Read the model definition and answer for the solid it produces. Units are mm, in the model's axes. Face numbers are marked on the shaded views. Coordinates: 2 decimals unless noted, no trailing zeros. Order: outer loops, then holes, each group sorted by start corner. A loop starts at its lowest first (then second) coordinate and runs counter-clockwise, first axis right, second up. Notation, with made-up numbers: (-2.5, -11.5) -> (2.5, -11.5) arc R10 ccw to (2.5, 3.5) -> close; hole circle Ø6 at (-18.5, 44.25). An arc over 180 degrees is marked (long way). Answer in a Markdown table with one row per item.
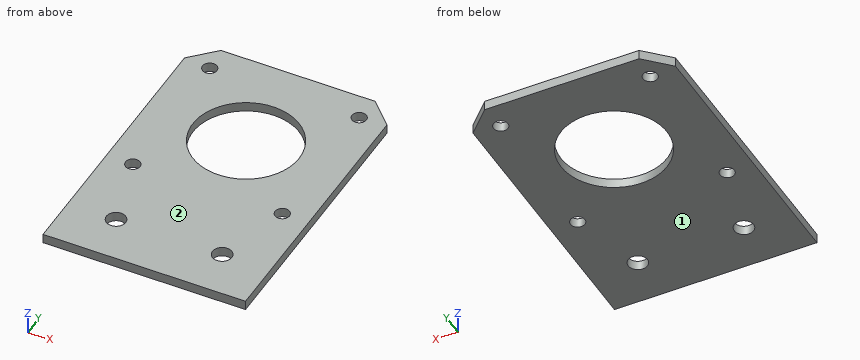
from build123d import *

# Parameters (mm, degrees)
F0_W     = 42
F0_H     = 62
F0_R     = 2
F0_R_2   = 1.5
F0_R_3   = 11
F1_DEPTH = 2
F2_SIZE  = 5


with BuildPart() as f1:
    # F0 (on Top) → F1 (new body)
    with BuildSketch(Plane.XY):
        Rectangle(F0_W, F0_H)
        with Locations((-11, -21)):
            Circle(F0_R, mode=Mode.SUBTRACT)
        with Locations((-15.5, -5.5)):
            Circle(F0_R_2, mode=Mode.SUBTRACT)
        with Locations((11, -21)):
            Circle(F0_R, mode=Mode.SUBTRACT)
        with Locations((15.5, -5.5)):
            Circle(F0_R_2, mode=Mode.SUBTRACT)
        with Locations((-15.5, 25.5)):
            Circle(F0_R_2, mode=Mode.SUBTRACT)
        with Locations((0, 10)):
            Circle(F0_R_3, mode=Mode.SUBTRACT)
        with Locations((15.5, 25.5)):
            Circle(F0_R_2, mode=Mode.SUBTRACT)
    extrude(amount=F1_DEPTH)

    # F2
    f2_edges = [f1.edges().sort_by_distance(p)[0] for p in [
        (21, 31, 1),
        (-21, 31, 1),
    ]]
    chamfer(f2_edges, length=F2_SIZE)


solid = f1.part
Q1. For a pull along Z with two mould halves and no side action, classify the marked faces 1 and 2 as pulls with the +Z half, pulls with the -Z half, needs draft (parallel to the pull), parting line crosses it, or undercut.
Outcome:
| item | result |
|---|---|
| face 1 | pulls with the -Z half |
| face 2 | pulls with the +Z half |
Q2. The part is cut by section B-B (y = 10). Write down the section's boundary in (x, z).
Outcome:
| item | result |
|---|---|
| outline | (-21, 0) -> (-11, 0) -> (-11, 2) -> (-21, 2) -> close; (11, 0) -> (21, 0) -> (21, 2) -> (11, 2) -> close |
Q3. The part is cut by section C-C (x = -2.5). Write down the section's boundary in (y, z), then the cut area to 3 significant figures.
Outcome:
| item | result |
|---|---|
| outline | (-31, 0) -> (-0.71, 0) -> (-0.71, 2) -> (-31, 2) -> close; (20.71, 0) -> (31, 0) -> (31, 2) -> (20.71, 2) -> close |
| area | 81.2 mm² |
Q4. Given pin 1 (2.5 mm diameter, centred on x = 15.5, y = 25.5, fed in from -Z), flat-ended and moving along its own axis, determine where the tip first touches the part or whether it passes through.
Outcome:
| item | result |
|---|---|
| pin 1 | through |
Q5. Consider line 1 (Y direction, x = -15.5, z = 0.5); line 2 (Y direction, x = 16.5, z = 0.4); line 3 (X direction, y = -20.5, z = 1). Determine where each line is inside the solid, lowest interval first.
Outcome:
| item | result |
|---|---|
| line 1 | -31 to -7, -4 to 24, 27 to 31 |
| line 2 | -31 to -6.62, -4.38 to 24.38, 26.62 to 30.5 |
| line 3 | -21 to -12.94, -9.06 to 9.06, 12.94 to 21 |
Q6. The part is cut by section D-D (z = 1.35). Write down the section's boundary in (x, y), then the cut area to 3 significant figures.
Outcome:
| item | result |
|---|---|
| outline | (-21, -31) -> (21, -31) -> (21, 26) -> (16, 31) -> (-16, 31) -> (-21, 26) -> close; hole circle Ø3 at (-15.5, -5.5); hole circle Ø3 at (-15.5, 25.5); hole circle Ø4 at (-11, -21); hole circle Ø22 at (0, 10); hole circle Ø4 at (11, -21); hole circle Ø3 at (15.5, -5.5); hole circle Ø3 at (15.5, 25.5) |
| area | 2,150 mm² |
Q7. The part is cut by section A-A (y = -5.5). Write down the section's boundary in (x, z).
Outcome:
| item | result |
|---|---|
| outline | (-21, 0) -> (-17, 0) -> (-17, 2) -> (-21, 2) -> close; (-14, 0) -> (14, 0) -> (14, 2) -> (-14, 2) -> close; (17, 0) -> (21, 0) -> (21, 2) -> (17, 2) -> close |
